```python
from build123d import *

# Parameters (mm, degrees)
SKETCH_1_R          = 22
EXTRUDE_1_DEPTH     = 0.6
SKETCH_2_R          = 3.25
CUT_EXTRUDE_1_DEPTH = 32.118483254
SKETCH_3_R          = 1.5
CUT_EXTRUDE_2_DEPTH = 32.118483254
SKETCH_5_W          = 56.096765119
SKETCH_5_H          = 19.515049226
SKETCH_5_W_2        = 56.672855133
SKETCH_5_H_2        = 21.675386779
CUT_EXTRUDE_4_DEPTH = 32.118483254
FILLET_1_R          = 5


with BuildPart() as part:
    # Эскиз1 → Бобышка-Вытянуть1 (new body)
    with BuildSketch(Plane.XY):
        Circle(SKETCH_1_R)
    extrude(amount=EXTRUDE_1_DEPTH)

    # Эскиз2 → Вырез-Вытянуть1 (cut, through all)
    with BuildSketch(Plane.XY.offset(0.6)):
        Circle(SKETCH_2_R)
    extrude(amount=-CUT_EXTRUDE_1_DEPTH, mode=Mode.SUBTRACT)

    # Эскиз3 → Вырез-Вытянуть2 (cut, through all)
    with BuildSketch(Plane.XY.offset(0.6)):
        with Locations((-15, 0)):
            Circle(SKETCH_3_R)
        with Locations((15, 0)):
            Circle(SKETCH_3_R)
    extrude(amount=-CUT_EXTRUDE_2_DEPTH, mode=Mode.SUBTRACT)

    # Эскиз5 → Вырез-Вытянуть4 (cut, through all)
    with BuildSketch(Plane.XY.offset(0.6)):
        with Locations((0.108016877, 18.757524613)):
            Rectangle(SKETCH_5_W, SKETCH_5_H)
        with Locations((0.396061884, -20.83769339)):
            Rectangle(SKETCH_5_W_2, SKETCH_5_H_2)
    extrude(amount=-CUT_EXTRUDE_4_DEPTH, mode=Mode.SUBTRACT)

    # Скругление1
    fillet_1_edges = [part.edges().sort_by_distance(p)[0] for p in [
        (-20.0748599, 9, 0.3),
        (20.0748599, 9, 0.3),
        (19.595917942, -10, 0.3),
        (-19.595917942, -10, 0.3),
    ]]
    fillet(fillet_1_edges, radius=FILLET_1_R)


solid = part.part
```
Source: CAD feature listing. Evaluate the final solid. Frame: model axes, mm. Give positions to 0.01 mm unless a question says otherwise; leave off trailing zeros. Loops run counter-clockwise (first coordinate to the right, second up) from the corner with the lowest first, then second, coordinate; pieces in that order, holes last. Notation, with made-up numbers: (69.25, 84) - (97.25, 84) arc R32 cw to (97.25, 121) - close; hole circle Ø10 at (75, 8). An arc over 180 degrees is marked (long way). Use CSV: the item, a comma, the result in double quotes. Start each with the question number.
1. Section B-B (y = 0). Output: boundary loops of the cut face in (x, z).
2. Draft query along X for faces 1 (the cylindrical face through (-16.5, 0.07, 0.3)), 2 (the flat face through (0, 4, 0)), 3 (the cylindrical face through (-21.992, -0.588, 0.296)). Return one class per face: +X half, -X half, draft (parallel to the pull), parting line (faces both ways), or undercut.
3. Section A-A (x = 0). Output: boundary loops of the cut face in (y, z), then the cut area to 3 significant figures.
4. Section C-C (z = 0.4). Output: boundary loops of the cut face in (x, y), then the cut area to 3 significant figures.
5. Section D-D (y = 2.5). Output: boundary loops of the cut face in (x, z).
6. Ray query, L1, parallel to Y at x = 0, z = 0.4; L2, parallel to Y at x = -15, z = 0.4; L3, parallel to X at y = -2.5, z = 0.45. Return the intervals inside material, ascending.
Response:
1,outline,"(-22, 0) - (-16.5, 0) - (-16.5, 0.6) - (-22, 0.6) - close; (-13.5, 0) - (-3.25, 0) - (-3.25, 0.6) - (-13.5, 0.6) - close; (3.25, 0) - (13.5, 0) - (13.5, 0.6) - (3.25, 0.6) - close; (16.5, 0) - (22, 0) - (22, 0.6) - (16.5, 0.6) - close"
2,face 1,"undercut"
2,face 2,"draft"
2,face 3,"-X half"
3,outline,"(-10, 0) - (-3.25, 0) - (-3.25, 0.6) - (-10, 0.6) - close; (3.25, 0) - (9, 0) - (9, 0.6) - (3.25, 0.6) - close"
3,area,"7.50 mm²"
4,outline,"(-21.38, 5.18) arc R22 ccw to (-21.03, -6.47) arc R5 ccw to (-16.25, -10) - (16.25, -10) arc R5 ccw to (21.03, -6.47) arc R22 ccw to (21.38, 5.18) arc R5 ccw to (16.52, 9) - (-16.52, 9) arc R5 ccw to start; hole circle Ø3 at (-15, 0); hole circle Ø6.5 at (0, 0); hole circle Ø3 at (15, 0)"
4,area,"752 mm²"
5,outline,"(-21.86, 0) - (-2.08, 0) - (-2.08, 0.6) - (-21.86, 0.6) - close; (2.08, 0) - (21.86, 0) - (21.86, 0.6) - (2.08, 0.6) - close"
6,L1,"-10 to -3.25, 3.25 to 9"
6,L2,"-10 to -1.5, 1.5 to 9"
6,L3,"-21.86 to -2.08, 2.08 to 21.86"
